Could you check a few things on this model? Use its own coordinates, in mm. A direction names the side the tool comes from. Coordinates: 2 decimals unless noted, no trailing zeros. Write each loop counter-clockwise with the first axis right and the second up, starting at its lowest first coordinate (ties: lowest second). Pieces come first, ordered by that corner, then holes. Notation, with made-up numbers: M 69.25,46 L 108.25,46 A11 ccw 108.25,54 Z; hole C -1,55 d10. An arc over 180 degrees is marked long. Write item = value, one per line.
```python
from build123d import *

# Parameters (mm, degrees)
SKETCH1_R           = 3.5
BOSS_EXTRUDE1_DEPTH = 34.2
SKETCH2_R           = 9.45299319
BOSS_EXTRUDE2_DEPTH = 5
CUT_EXTRUDE1_DEPTH  = 1.92
SKETCH4_R           = 1
CUT_EXTRUDE2_DEPTH  = 10


with BuildPart() as part:
    # Sketch1 → Boss-Extrude1 (new body)
    with BuildSketch(Plane.XY):
        Circle(SKETCH1_R)
    extrude(amount=BOSS_EXTRUDE1_DEPTH)

    # Sketch2 → Boss-Extrude2 (add)
    with BuildSketch(Plane.XY.offset(34.2)):
        Circle(SKETCH2_R)
    extrude(amount=BOSS_EXTRUDE2_DEPTH)

    # Sketch3 → Cut-Extrude1 (cut)
    with BuildSketch(Plane(origin=(0, 0, 0), x_dir=(-1, 0, 0), z_dir=(0, 0, -1))):
        Polygon((-1.943409889, 1.572627739), (-2.333640517, -0.896728464), (-0.390230628, -2.469356203), (1.943409889, -1.572627739), (2.333640517, 0.896728464), (0.390230628, 2.469356203), align=None)
    extrude(amount=-CUT_EXTRUDE1_DEPTH, mode=Mode.SUBTRACT)

    # Sketch4 → Cut-Extrude2 (cut)
    with BuildSketch(Plane(origin=(0, 0, 1.92), x_dir=(-1, 0, 0), z_dir=(0, 0, -1))):
        Circle(SKETCH4_R)
    extrude(amount=-CUT_EXTRUDE2_DEPTH, mode=Mode.SUBTRACT)


solid = part.part
```
Item 1: Imagine slicing it at A-A (x = 0). Write out the boundary of the cut face in (y, z).
Numbers:
outline = M -9.45,34.2 L -3.5,34.2 L -3.5,0 L -2.32,0 L -2.32,1.92 L -1,1.92 L -1,11.92 L 1,11.92 L 1,1.92 L 2.32,1.92 L 2.32,0 L 3.5,0 L 3.5,34.2 L 9.45,34.2 L 9.45,39.2 L -9.45,39.2 Z
Item 2: For faces 1 (the face through (0, 0, 39.2)), 2 (the face through (0.76, 2.027, 0.947)), which set-ups out of +Z, -Z, +X, -X, +Y, -Y let a thin tool reach every point of the face, with its end or its side?
Numbers:
face_1 = +Z, +X, -X, +Y, -Y
face_2 = -Z
Item 3: Imagine slicing it at D-D (x = -7). Write out the boundary of the cut face in (y, z), and give its area (3 significant figures).
Numbers:
outline = M -6.35,34.2 L 6.35,34.2 L 6.35,39.2 L -6.35,39.2 Z
area = 63.5 mm²
Item 4: I'm going to push flat-ended pins straight in: P1, Ø8, axis at x = -6.5, y = -6.5, coming from the -Z side; P2, Ø3, axis at x = 0, y = 0, coming from the -Z side; P3, Ø3, axis at x = -4, z = 8.5, coming from the -Y side. Where does each tip first touch, or does it pass through?
Numbers:
P1 = 34.2
P2 = 1.92
P3 = -2.45
Item 5: Imagine slicing it at C-C (z = 17.5). Write out the boundary of the cut face in (x, y).
Numbers:
outline = C 0,0 d7
Item 6: If I drill on line 1 along Y through (x, z) = (0, 5.25); line 2 along Z through (x, y) = (2.25, 7); line 3 along X through (y, z) = (-0.5, 12.5), over which ranges is the centre line in solid material (lowest first)?
Numbers:
line_1 = -3.5 to -1, 1 to 3.5
line_2 = 34.2 to 39.2
line_3 = -3.46 to 3.46
Item 7: If we mould it in two halves opening along X, with no side actions, what happens to faces 3 (the face through (-1, -1, 1.92)), 4 (the face through (0, -4, 34.2)), 5 (the face through (-2.05, -9.23, 36.67))? For each: pulls with the +X half, pulls with the -X half, needs draft (parallel to the pull), parting line crosses it, or undercut.
Numbers:
face_3 = undercut
face_4 = needs draft
face_5 = parting line crosses it
Item 8: Imagine slicing it at B-B (y = 0). Write out the boundary of the cut face in (x, z), and give its area (3 significant figures).
Numbers:
outline = M -9.45,34.2 L -3.5,34.2 L -3.5,0 L -2.19,0 L -2.19,1.92 L -1,1.92 L -1,11.92 L 1,11.92 L 1,1.92 L 2.19,1.92 L 2.19,0 L 3.5,0 L 3.5,34.2 L 9.45,34.2 L 9.45,39.2 L -9.45,39.2 Z
area = 306 mm²
